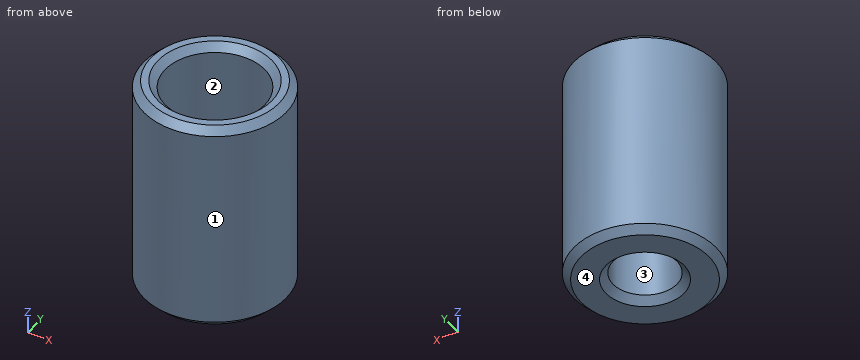
from build123d import *

# Parameters (mm, degrees)
F0_W     = 31.75
F0_H     = 95.25
F2_R     = 22.225
F3_DEPTH = 50.8
F4_R     = 14.2875
F5_DEPTH = 95.251
F6_SIZE  = 3.175


with BuildPart() as f1:
    # F0 (on Front) → F1 (revolve)
    with BuildSketch(Plane.XZ):
        with Locations((15.875, 47.625)):
            Rectangle(F0_W, F0_H)
    revolve(axis=Axis((0, 0, 30.3924912523), (0, 0, 1)))

    # F2 (on face) → F3 (cut)
    with BuildSketch(Plane.XY.offset(95.25)):
        Circle(F2_R)
    extrude(amount=-F3_DEPTH, mode=Mode.SUBTRACT)

    # F4 (on face) → F5 (cut, through all)
    with BuildSketch(Plane(origin=(0, 0, 0), x_dir=(1, 0, 0), z_dir=(0, 0, -1))):
        Circle(F4_R)
    extrude(amount=-F5_DEPTH, mode=Mode.SUBTRACT)

    # F6
    f6_edges = [f1.edges().sort_by_distance(p)[0] for p in [
        (-31.75, 0, 0),
        (-31.75, 0, 95.25),
        (-22.225, 0, 95.25),
        (-14.2875, 0, 44.45),
        (-14.2875, 0, 0),
        (14.2875, 0, 22.225),
    ]]
    chamfer(f6_edges, length=F6_SIZE)


solid = f1.part
Work out the finished part from the listing and answer in its coordinate system (mm). Face numbers are marked on the shaded views. Give positions to 0.01 mm unless a question says otherwise; leave off trailing zeros. Loops run counter-clockwise (first coordinate to the right, second up) from the corner with the lowest first, then second, coordinate; pieces in that order, holes last. Notation, with made-up numbers: (57, -30.75) -> (78, -30.75) arc R21 ccw to (78, -11.75) -> close; hole circle Ø5 at (80.5, 7.25). An arc over 180 degrees is marked (long way). Use a Markdown table: item, result. Add a question column.
1) Consider line 1 along Y through (x, z) = (0, 65.5) (3 decimals); line 2 along Y through (x, z) = (0, 20); line 3 along X through (y, z) = (1, 66). Determine where each line is inside the solid, lowest interval first.
2) For a pull along X with two mould halves and no side action, classify the marked faces 1, 2, 3 and 4 as +X half, -X half, draft (parallel to the pull), parting line (faces both ways), or undercut.
3) Each of these flat-tipped pins is pushed along its axis until it touches: P1, Ø4, axis at x = -4, z = 53.5, coming from the -Y side; P2, Ø1, axis at x = -20, z = 84.5, coming from the -Y side; P3, Ø2, axis at y = 15.5, z = 26.5, coming from the -X side; P4, Ø1.5, axis at x = -22.5, y = -12, coming from the -Z side. Where does it stop, or does it pass through?
4) The part is cut by section C-C, the plane z = 46. Determine the outline of the cut face in (x, y) (3 decimals).
Reported:
| question | item | result |
|---|---|---|
| 1 | line 1 | y = -31.75 to -22.225, 22.225 to 31.75 |
| 1 | line 2 | y = -31.75 to -14.29, 14.29 to 31.75 |
| 1 | line 3 | x = -31.73 to -22.2, 22.2 to 31.73 |
| 2 | face 1 | parting line |
| 2 | face 2 | undercut |
| 2 | face 3 | undercut |
| 2 | face 4 | draft |
| 3 | P1 | stops at y = -31.69 |
| 3 | P2 | stops at y = -25.06 |
| 3 | P3 | stops at x = -28.25 |
| 3 | P4 | stops at z = 0 |
| 4 | outline | circle Ø63.5 at (0, 0); hole circle Ø44.45 at (0, 0) |
